Build history of the part. All positions in model axes, mm. A direction names the side the tool comes from. Round coordinates to 2 decimals unless told otherwise and drop trailing zeros. Write each loop counter-clockwise with the first axis right and the second up, starting at its lowest first coordinate (ties: lowest second). Pieces come first, ordered by that corner, then holes. Notation, with made-up numbers: (-29.75, 47.5) -> (-16.75, 47.5) arc R21 cw to (-16.75, 51.5) -> close; hole circle Ø5 at (21, 54). An arc over 180 degrees is marked (long way). Return JSON: item names as keys, results as strings.
Solid Edge part; units mm, degrees
sketch "Sketch1" plane through (0, 0, 0) normal (0, 0, 1) x (1, 0, 0)
  circle A0 centre (0, 0) radius 13.125
extrude "Protrusion1" add sketch "Sketch1" along normal blind 9
sketch "Sketch2" plane through (0, 0, 9) normal (0, 0, 1) x (1, 0, 0)
  circle A0 centre (0, 0) radius 11.1
extrude "ExtrudedCutout_1" cut sketch "Sketch2" against normal blind 7
sketch "Sketch3" plane through (0, 0, 0) normal (0, 0, -1) x (0, -1, 0)
  circle A0 centre (0, 0) radius 8
extrude "Cutout1" cut sketch "Sketch3" against normal through all
sketch "Sketch4" plane through (0, 0, 0) normal (0, 0, -1) x (0, -1, 0)
  circle A0 centre (0, 0) radius 11.1
  circle A1 centre (0, 0) radius 13.125
extrude "ExtrudedProtrusion_3" add sketch "Sketch4" along normal blind 7
chamfer "Chamfer_1" distance 6 angle 45 1 edges at (0, 11.1, 0)
Q1. Saw through at D-D on z = -2.25. List the corners of the cut face in (x, y) (3 decimals), then the cut area to 3 significant figures.
Verdict:
{"outline": "circle Ø26.25 at (0, 0); hole circle Ø16 at (0, 0)", "area": "340 mm²"}
Q2. Saw through at A-A on y = 0. List the corners of the cut face in (x, z) (3 decimals).
Verdict:
{"outline": "(-13.125, -7) -> (-11.1, -7) -> (-11.1, -6) -> (-8, -2.9) -> (-8, 2) -> (-11.1, 2) -> (-11.1, 9) -> (-13.125, 9) -> close; (8, -2.9) -> (11.1, -6) -> (11.1, -7) -> (13.125, -7) -> (13.125, 9) -> (11.1, 9) -> (11.1, 2) -> (8, 2) -> close"}
Q3. 3-axis set-ups, long thin cutter, end or side, ignore diameter. For faces 4 (the cylindrical face through (5.97, 9.36, 5.55)), 5 (the flat face through (11, 3, -7)), 6 (the cylindrical face through (9.36, -5.97, -6.49)): which of +Z, -Z, +X, -X, +Y, -Y reach the whole face in a straight line?
Verdict:
{"face 4": "+Z", "face 5": "-Z, +X, -X, +Y, -Y", "face 6": "-Z"}
Q4. Two-plate mould, pull along Y, no slides. Class faces 1 (the flat face through (-11, 3, 9)), 2 (the conical face through (8, 1.8, -3.1)), 3 (the cylindrical face through (4.885, -12.182, -0.666)): +Y half, -Y half, draft (parallel to the pull), parting line (faces both ways), or undercut.
Verdict:
{"face 1": "draft", "face 2": "undercut", "face 3": "parting line"}
Q5. Pin check, flat tips, straight feed: pin 1 Ø13 at (x, y) = (0, 0) entering from -Z; pin 2 Ø6 at (y, z) = (1.5, 2) entering from +X (3 decimals); pin 3 Ø1.5 at (x, z) = (-1.5, 7) entering from +Y; pin 4 Ø3 at (y, z) = (5.5, 1) entering from +X. Stop position of each tip, or through.
Verdict:
{"pin 1": "passes through", "pin 2": "stops at x = 13.125", "pin 3": "stops at y = 13.1", "pin 4": "stops at x = 12.5"}
Q6. Saw through at C-C on z = -5.25. List the corners of the cut face in (x, y) (3 decimals), then the cut area to 3 significant figures.
Verdict:
{"outline": "circle Ø26.25 at (0, 0); hole circle Ø20.7 at (0, 0)", "area": "205 mm²"}
Q7. Wall check: L1, parallel to Y at x = 0, z = 6.5 (3 decimals); L2, parallel to Y at x = 0, z = -0.75 (3 decimals). Give the ranges that are in metal, low to high.
Verdict:
{"L1": "y = -13.125 to -11.1, 11.1 to 13.125", "L2": "y = -13.125 to -8, 8 to 13.125"}
